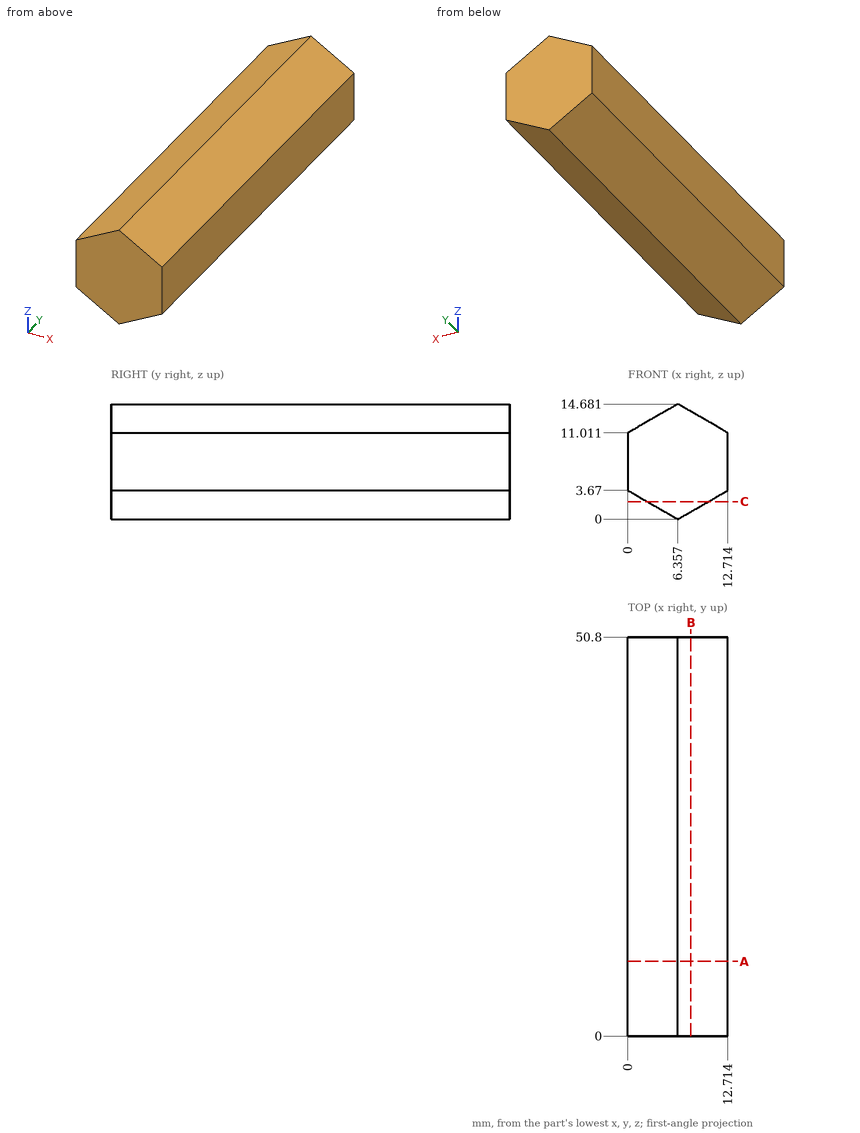
Job drawing, mm, ordinate dimensions from the low corner. One solid piece. Round coordinates to 2 decimals unless told otherwise and drop trailing zeros. Order: outer loops, then holes, each group sorted by start corner. A loop starts at its lowest first (then second) coordinate and runs counter-clockwise, first axis right, second up. Notation, with made-up numbers: (30, -4) -> (43, -4) arc R26 cw to (43, 18) -> close; hole circle Ø2 at (58, -21). An arc over 180 degrees is marked (long way). Write item = value, one per line.
(1) Flat gauge pins, fed straight in: P1, Ø5, axis at x = 5.5, y = 36, coming from the -Z side; P2, Ø4, axis at x = 9, y = 6.5, coming from the -Z side. Where does each tip first touch, or does it go through?
Answers follow:
P1 = 0
P2 = 0.37
(2) Drill centre lines: L1, parallel to X at y = 30.5, z = 14.25 (1 decimal); L2, parallel to Z at x = 11.25, y = 23 (1 decimal); L3, parallel to X at y = 18, z = 13.5 (1 decimal). Where is each one in solid material? Low to high.
Answers follow:
L1 = 5.6 to 7.1
L2 = 2.8 to 11.9
L3 = 4.3 to 8.4
(3) Cut at A-A (y = 9.5). Write the cut outline in (x, z).
Answers follow:
outline = (0, 3.67) -> (6.36, 0) -> (12.71, 3.67) -> (12.71, 11.01) -> (6.36, 14.68) -> (0, 11.01) -> close
(4) Cut at C-C (z = 2.25). Write the cut outline in (x, y), plus the area to 3 significant figures.
Answers follow:
outline = (2.46, 0) -> (10.25, 0) -> (10.25, 50.8) -> (2.46, 50.8) -> close
area = 396 mm²
(5) Cut at B-B (x = 8). Write the cut outline in (y, z).
Answers follow:
outline = (0, 0.95) -> (50.8, 0.95) -> (50.8, 13.73) -> (0, 13.73) -> close
